The drawing under review shows one solid part. Ordinate dimensions are in mm from its lowest x, y, z. A direction names the side the tool comes from. Round coordinates to 2 decimals unless told otherwise and drop trailing zeros. Write each loop counter-clockwise with the first axis right and the second up, starting at its lowest first coordinate (ties: lowest second). Pieces come first, ordered by that corner, then holes. Notation, with made-up numbers: M 34,82.25 L 80,82.25 A20 cw 80,109.25 Z; hole C 26,49.25 d4. An arc over 180 degrees is marked long. Write item = value, one per line. Start each with the question number.
Item 1: Take a section at A-A, the plane y = 4. Give the boundary of the cut face in (x, z) (1 decimal).
Item 2: Take a section at B-B, the plane x = 4. Give the boundary of the cut face in (y, z).
Item 3: To check wall thickness, follow line 1 along X through (y, z) = (4, 5.55); line 2 along Y through (x, z) = (4, 5.35); line 3 along X through (y, z) = (4, 3.75). State the ranges of each line that lie inside material, in increasing order.
Item 4: Take a section at C-C, the plane z = 5.25. Give the boundary of the cut face in (x, y) (1 decimal).
Item 5: For pin 1 Ø0.8 at (x, y) = (3.5, 4) entering from +Z; pin 2 Ø3 at (x, y) = (13.5, 2) entering from -Z; pin 3 Ø1 at (y, z) = (2.5, 2) entering from +X, all flat-tipped, find the tip position at first contact; note any pin that passes through.
Item 6: Tool access review of the marked faces 1 and 2: name each direction out of +Z, -Z, +X, -X, +Y, -Y from which nothing blocks a thin tool from reaching the whole face with its end or side.
Item 7: Take a section at D-D, the plane z = 1.5. Give the boundary of the cut face in (x, y).
Item 8: The part is to be moulded in two halves that separate along Y. For the marked faces 3, 4 and 5, say which applies: +Y half, -Y half, draft (parallel to the pull), parting line (faces both ways), or undercut.
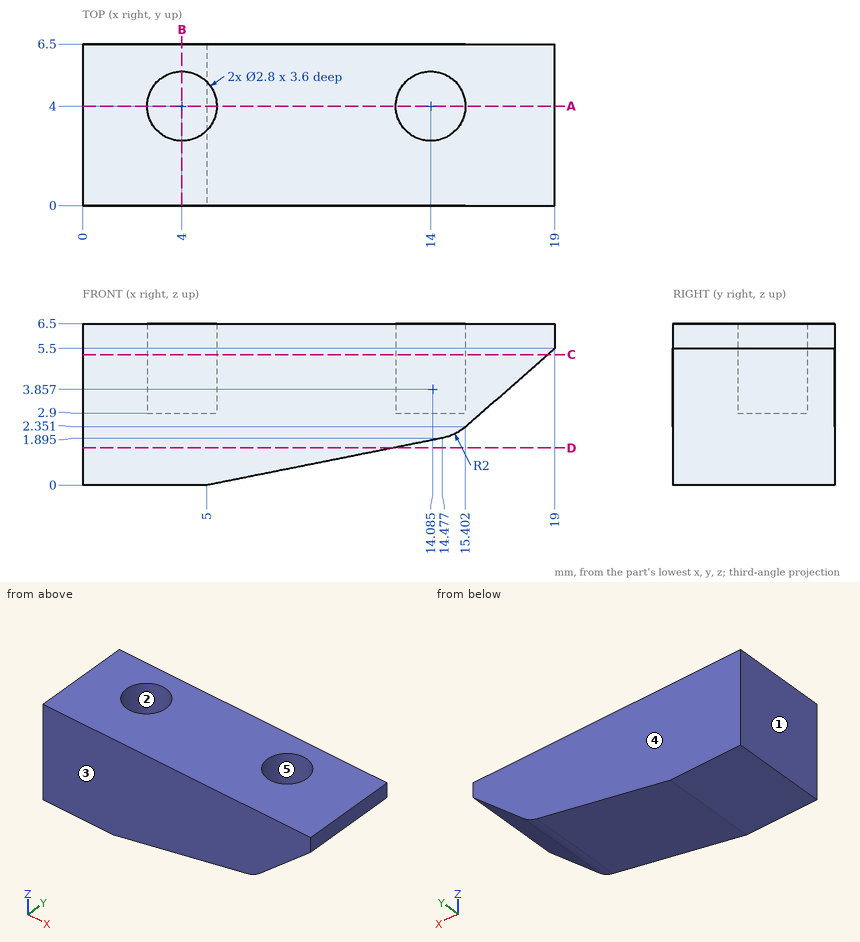
Response values:
q1.outline = M 0,0 L 5,0 L 14.5,1.9 A2 ccw 15.4,2.4 L 19,5.5 L 19,6.5 L 15.4,6.5 L 15.4,2.9 L 12.6,2.9 L 12.6,6.5 L 5.4,6.5 L 5.4,2.9 L 2.6,2.9 L 2.6,6.5 L 0,6.5 Z
q2.outline = M 0,0 L 6.5,0 L 6.5,6.5 L 5.4,6.5 L 5.4,2.9 L 2.6,2.9 L 2.6,6.5 L 0,6.5 Z
q3.line_1 = 0 to 2.6, 5.4 to 12.6, 15.4 to 19
q3.line_2 = 0 to 2.6, 5.4 to 6.5
q3.line_3 = 0 to 2.6, 5.4 to 12.6, 15.4 to 17
q4.outline = M 0,0 L 18.7,0 L 18.7,6.5 L 0,6.5 Z; hole C 4,4 d2.8; hole C 14,4 d2.8
q5.pin_1 = 2.9
q5.pin_2 = 1.4
q5.pin_3 = 15.57
q6.face_1 = +Z, -Z, -X, +Y, -Y
q6.face_2 = +Z
q7.outline = M 0,0 L 12.5,0 L 12.5,6.5 L 0,6.5 Z
q8.face_3 = -Y half
q8.face_4 = +Y half
q8.face_5 = undercut
